Autodesk Inventor part; units mm, degrees
ref_plane "YZ Plane" through (0, 0, 0) normal (1, 0, 0) x (0, 1, 0)
ref_plane "XZ Plane" through (0, 0, 0) normal (0, 1, 0) x (-1, 0, 0)
ref_plane "XY Plane" through (0, 0, 0) normal (0, 0, 1) x (1, 0, 0)
sketch "Эскиз1" plane through (0, 0, 0) normal (0, 0, 1) x (1, 0, 0)
  circle A0 centre (5.6, 18) radius 0.52
  circle A1 centre (5.6, 18) radius 0.8
  line L0 (7.2, 17) -> (7.2, 18)
  line L1 (0, 36) -> (10, 36)
  line L2 (10, 36) -> (10, 34.5)
  line L3 (10, 34.5) -> (2, 34.5)
  line L4 (0, 0) -> (9.5856, 0)
  line L5 (0, 36) -> (0, 18)
  line L6 (0, 18) -> (2, 17.5)
  line L7 (2, 17.5) -> (5.6, 15)
  line L8 (5.6, 15) -> (7.2, 17)
  line L9 (5.6, 15) -> (0, 15) construction
  line L10 (0, 43.2) -> (0, -7.2)
  line L11 (-2, 0) -> (12, 0)
  line L12 (4.8, 18) -> (2, 18.7)
  line L13 (2, 18.7) -> (2, 34.5)
  line L14 (7.2, 18) -> (6.4, 18)
  dimension "d0" = 72
  dimension "d1" = 34
  dimension "d2" = 1.5
  dimension "d3" = 1.04
  dimension "d4" = 1.6
  dimension "d5" = 30
  dimension "d6" = 35
  dimension "d7" = 36
  dimension "d8" = 5.6
  dimension "d9" = 7.2
  dimension "d10" = 10
  dimension "d12" = 2
revolve "Базовый элемент" add sketch "Эскиз1" angle 360 about axis through (0, 0, 0) along (1, 0, 0) contours L14 L0 L8 L7 L6 L5 L1 L2 L3 L13 L12 A1
revolve "Пружинные1" add sketch "Эскиз1" angle 360 about axis through (0, 0, 0) along (1, 0, 0) contours A0 | A1
fillet "Сопряжение1" radius 0.4 3 edges at (10, -36, 0) (2, -34.5, 0) (0, -36, 0)
equation "\"d0\" = SD2"
equation "\"d3\" = SPDI"
equation "\"d4\" = SPDA"
equation "\"d8\" = SPDST"
equation "\"d9\" = SDI"
equation "\"d12\" = SD"
equation "\"d11\" = RR"
equation "\"SD2\" = 72"
equation "\"SWDT\" = 8"
equation "\"RR\" = 0.4"
equation "\"SD\" = 2"
equation "\"SPDA\" = 1.6"
equation "\"SPDI\" = 1.04"
equation "\"TKDM\" = 53"
equation "\"HLDM\" = 54.8"
equation "\"ABDM\" = 52"
equation "\"SDI\" = 7.2"
equation "\"SPDST\" = 5.6"
equation "\"LAB\" = 0.4"
properties part number "Манжет 1-50x72x8 ГОСТ 8752-79" material "Резина"
CAD build for the part. Positions are in the model's coordinates, mm. A direction names the side the tool comes from. Coordinates: 2 decimals unless noted, no trailing zeros. Use CSV: the item, a comma, the result in double quotes. Start each with the question number.
Q1. 3-axis set-ups, long thin cutter, end or side, ignore diameter. For faces 1 (the flat face through (7.2, 16, -7)), 2 (the conical face through (5.37, 14.46, -4.55)): which of +Z, -Z, +X, -X, +Y, -Y reach the whole face in a straight line?
Q2. Two-plate mould, pull along Y, no slides. Class faces 3 (the cylindrical face through (5.064, -4.686, 35.694)), 4 (the conical face through (4.625, 8.326, 16.008)), 5 (the flat face through (0, -8.4, 16.3)): +Y half, -Y half, draft (parallel to the pull), parting line (faces both ways), or undercut.
Q3. Probe probe 1 along Y at (x, z) = (5.75, 1); probe 2 along Y at (x, z) = (4.5, 16); probe 3 along Y at (x, z) = (5, 7). List the from-to ranges inside material, lowest first. Write a range as from..to.
Q4. Drop flat-ended pins along their axis: P1, Ø5, axis at x = 9, y = -22.5, coming from the +Z side; P2, Ø12, axis at y = -7.5, z = 6.5, coming from the -X side; P3, Ø2, axis at x = 7.5, y = 8.5, coming from the -Z side; P4, Ø10, axis at y = -15, z = 7.5, coming from the -X side. Give the stop position or say it passes through.
Here are the results:
1,face 1,"+X"
1,face 2,"-X"
2,face 3,"parting line"
2,face 4,"undercut"
2,face 5,"draft"
3,probe 1,"-35.99..-34.49, -18.76..-15.15, 15.15..18.76, 34.49..35.99"
3,probe 2,"-32.25..-30.57, -8.41..8.41, 30.57..32.25"
3,probe 3,"-35.31..-33.78, -17.16..-13.74, 13.74..17.16, 33.78..35.31"
4,P1,"z = 29.93"
4,P2,"x = 4.27"
4,P3,"z = -35.21"
4,P4,"x = 0"
